Could you check a few things on this model? Use its own coordinates, in mm. A direction names the side the tool comes from. Round coordinates to 2 decimals unless told otherwise and drop trailing zeros. Write each loop counter-clockwise with the first axis right and the second up, starting at its lowest first coordinate (ties: lowest second). Pieces come first, ordered by that corner, then holes. Notation, with made-up numbers: (-10, -35) -> (4, -35) arc R18 cw to (4, -31) -> close; hole circle Ø5 at (57.5, -6). An arc over 180 degrees is marked (long way). One line per question, with ' | ' between items. Start each with the question number.
1. Imagine slicing it at C-C, the plane y = -82. List the corners of the cut face in (x, z) for me, and give its area (3 significant figures).
2. If I drill on line 1 along Y through (x, z) = (30, 7.25); line 2 along Z through (x, y) = (-7, -20); line 3 along X through (y, z) = (-17, 7.5), over which ranges is the centre line in solid material (lowest first)? Write a range as [from, to].
3. Imagine slicing it at A-A, the plane x = -85. List the corners of the cut face in (y, z) for me, and give its area (3 significant figures).
4. Imagine slicing it at B-B, the plane x = -50.5. List the corners of the cut face in (y, z) for me, and give its area (3 significant figures).
5. For faces 1 (the flat face through (25, -44, 10)), 2 (the flat face through (-75, -44, 0)), 3 (the flat face through (-28, -44, 10)), 4 (the flat face through (-28, -40, 37)), 5 (the flat face through (-65, -24, 36)), which set-ups out of +Z, -Z, +X, -X, +Y, -Y let a thin tool reach every point of the face, with its end or its side?
6. Imagine slicing it at D-D, the plane y = -70. List the corners of the cut face in (x, z) for me, and give its area (3 significant figures).
7. Thinking about a two-plate mould opening in X: for faces 6 (the cylindrical face through (-91, -20, 5)), 7 (the flat face through (-95, -44, 5)), 8 (the flat face through (-28, -90, 12)), 9 (the flat face through (0, -44, 5)), which applies, released by +X, released by -X, zero draft, split by the parting line, or undercut?
8. For pin 1 Ø12 at (y, z) = (-22, 21.5) entering from +X; pin 2 Ø8 at (x, z) = (-52, 48.5) entering from +Y; pin 3 Ø15 at (x, y) = (-79, -25) entering from +Z; pin 4 Ø5 at (x, z) = (-53, 56.5) entering from -Y, each with a flat end and sliding along its axis, tell me the tip position at first contact or that it passes through.
from build123d import *

# Parameters (mm, degrees)
F1_DEPTH  = 90
F2_R      = 6
F3_DEPTH  = 10
F4_R      = 6
F5_DEPTH  = 10
F6_R      = 6
F8_DEPTH  = 10
F7_R      = 6
F9_DEPTH  = 10
F10_R     = 10
F11_DEPTH = 75


with BuildPart() as f1:
    # F0 (on Front) → F1 (new body)
    with BuildSketch(Plane.XZ):
        Polygon((-95, 10), (-95, 0), (-55, 0), (-55, 10), (0, 10), (0, 0), (40, 0), (40, 10), (10, 10), (10, 20), (-65, 20), (-65, 10), align=None)
    extrude(amount=F1_DEPTH)

    # F2 (on face) → F3 (cut)
    with BuildSketch(Plane.XY.offset(10)):
        with Locations((-85, -70)):
            Circle(F2_R)
    extrude(amount=-F3_DEPTH, mode=Mode.SUBTRACT)

    # F4 (on face) → F5 (cut)
    with BuildSketch(Plane.XY.offset(10)):
        with Locations((30, -70)):
            Circle(F4_R)
    extrude(amount=-F5_DEPTH, mode=Mode.SUBTRACT)

    # F6 (on face) → F8 (cut)
    with BuildSketch(Plane.XY.offset(10)):
        with Locations((-85, -20)):
            Circle(F6_R)
    extrude(amount=-F8_DEPTH, mode=Mode.SUBTRACT)

    # F7 (on face) → F9 (cut)
    with BuildSketch(Plane.XY.offset(10)):
        with Locations((30, -20)):
            Circle(F7_R)
    extrude(amount=-F9_DEPTH, mode=Mode.SUBTRACT)

    # F10 (on face) → F11 (join, through all)
    with BuildSketch(Plane(origin=(-65, 0, 0), x_dir=(0, -1, 0), z_dir=(-1, 0, 0))):
        with BuildLine():
            Line((0, 55), (0, 20))
            Line((0, 20), (40, 20))
            Line((40, 20), (40, 55))
            ThreePointArc((40, 55), (20, 75), (0, 55))
        make_face()
        with Locations((20, 55)):
            Circle(F10_R, mode=Mode.SUBTRACT)
    extrude(amount=-F11_DEPTH)


solid = f1.part
Geometry results:
1) outline: (-95, 0) -> (-55, 0) -> (-55, 10) -> (0, 10) -> (0, 0) -> (40, 0) -> (40, 10) -> (10, 10) -> (10, 20) -> (-65, 20) -> (-65, 10) -> (-95, 10) -> close | area: 1,550 mm2
2) line 1: y = [-90, -76], [-64, -26], [-14, 0] | line 2: z = [10, 45], [65, 75] | line 3: x = [-95, -90.2], [-79.8, -55], [0, 24.8], [35.2, 40]
3) outline: (-90, 0) -> (-76, 0) -> (-76, 10) -> (-90, 10) -> close; (-64, 0) -> (-26, 0) -> (-26, 10) -> (-64, 10) -> close; (-14, 0) -> (0, 0) -> (0, 10) -> (-14, 10) -> close | area: 660 mm2
4) outline: (-90, 10) -> (0, 10) -> (0, 55) arc R20 ccw to (-40, 55) -> (-40, 20) -> (-90, 20) -> close; hole circle Ø20 at (-20, 55) | area: 2,610 mm2
5) face 1: +Z, +X, +Y, -Y | face 2: -Z, +X, -X, +Y, -Y | face 3: -Z, +Y, -Y | face 4: +Z, +X, -X, -Y | face 5: +Z, -X, +Y, -Y
6) outline: (-95, 0) -> (-91, 0) -> (-91, 10) -> (-95, 10) -> close; (-79, 0) -> (-55, 0) -> (-55, 10) -> (0, 10) -> (0, 0) -> (24, 0) -> (24, 10) -> (10, 10) -> (10, 20) -> (-65, 20) -> (-65, 10) -> (-79, 10) -> close; (36, 0) -> (40, 0) -> (40, 10) -> (36, 10) -> close | area: 1,310 mm2
7) face 6: undercut | face 7: released by -X | face 8: zero draft | face 9: undercut
8) pin 1: stops at x = 10 | pin 2: stops at y = 0 | pin 3: stops at z = 10 | pin 4: stops at y = -40
